from build123d import *

# Parameters (mm, degrees)
SKETCH1_R           = 6.33
BOSS_EXTRUDE1_DEPTH = 1.5
SKETCH2_R           = 20.2
BOSS_EXTRUDE2_DEPTH = 71
SKETCH6_R           = 6
BOSS_EXTRUDE4_DEPTH = 3
SKETCH7_R           = 2
BOSS_EXTRUDE5_DEPTH = 9
SKETCH8_R           = 1.65
CUT_EXTRUDE1_DEPTH  = 4


with BuildPart() as part:
    # Sketch1 → Boss-Extrude1 (new body)
    with BuildSketch(Plane.XY):
        Circle(SKETCH1_R)
    extrude(amount=BOSS_EXTRUDE1_DEPTH)

    # Sketch2 → Boss-Extrude2 (add)
    with BuildSketch(Plane.XY):
        Circle(SKETCH2_R)
    extrude(amount=-BOSS_EXTRUDE2_DEPTH)

    # Sketch6 → Boss-Extrude4 (add)
    with BuildSketch(Plane(origin=(0, 0, -71), x_dir=(-1, 0, 0), z_dir=(0, 0, -1))):
        Circle(SKETCH6_R)
    extrude(amount=BOSS_EXTRUDE4_DEPTH)

    # Sketch7 → Boss-Extrude5 (add)
    with BuildSketch(Plane(origin=(0, 0, -74), x_dir=(-1, 0, 0), z_dir=(0, 0, -1))):
        Circle(SKETCH7_R)
    extrude(amount=BOSS_EXTRUDE5_DEPTH)

    # Sketch8 → Cut-Extrude1 (cut)
    with BuildSketch(Plane(origin=(0, 0, -71), x_dir=(-1, 0, 0), z_dir=(0, 0, -1))):
        with Locations((-12.5, 0)):
            Circle(SKETCH8_R)
        with Locations((12.5, 0)):
            Circle(SKETCH8_R)
    extrude(amount=-CUT_EXTRUDE1_DEPTH, mode=Mode.SUBTRACT)


solid = part.part
Can you work these out from the model? Positions are in its coordinate system, mm. A direction names the side the tool comes from. Give positions to 0.01 mm unless a question says otherwise; leave off trailing zeros. Order: outer loops, then holes, each group sorted by start corner. A loop starts at its lowest first (then second) coordinate and runs counter-clockwise, first axis right, second up. Notation, with made-up numbers: M -16,75 L 4,75 A19 cw 4,89 Z; hole C 21.25,16 d3. An arc over 180 degrees is marked long. Use a Markdown table: item, result. Add a question column.
Item 1: Suppose I cut it at C-C (z = -52). List the corners of the cut face in (x, y) for me, then the cut area to 3 significant figures.
Item 2: Will these pins go through, and if not, where does the flat tip stop? pin 1 (12 mm diameter, centred on x = 7.5, y = 2, fed in from -Z); pin 2 (3 mm diameter, centred on x = -12.5, y = 0, fed in from +Z); pin 3 (4 mm diameter, centred on x = -1.5, z = -70, fed in from +Y); pin 4 (8 mm diameter, centred on y = -6.5, z = -69.5, fed in from -X).
Item 3: If I drill on L1, parallel to Z at x = 0, y = 15.5; L2, parallel to Y at x = 12.5, z = -68.85; L3, parallel to Y at x = -10, z = -59.5, over which ranges is the centre line in solid material (lowest first)? Write a range as [from, to].
Item 4: Suppose I cut it at B-B (y = 0). List the corners of the cut face in (x, z) for me, then the cut area to 3 significant figures.
Item 5: We'd pull the mould along X, two halves only. Please class faces 1 (the flat face through (-3, 0, -74)), 2 (the cylindrical face through (6, 0, -72)), 3 (the cylindrical face through (10.976, -0.632, -69.028)): +X half, -X half, draft (parallel to the pull), parting line (faces both ways), or undercut.
Item 6: Suppose I cut it at A-A (x = 0). List the corners of the cut face in (y, z) for me.
Item 7: For faces 4 (the flat face through (-5, 5, 0)), 5 (the flat face through (0, 0, -83)), 6 (the flat face through (13, 0, -67)), which set-ups out of +Z, -Z, +X, -X, +Y, -Y let a thin tool reach every point of the face, with its end or its side?
Item 8: Suppose I cut it at D-D (x = 12.5). List the corners of the cut face in (y, z) for me, then the cut area to 3 significant figures.
Answer sheet:
| question | item | result |
|---|---|---|
| 1 | outline | C 0,0 d40.4 |
| 1 | area | 1,280 mm² |
| 2 | pin 1 | stops at z = -83 |
| 2 | pin 2 | stops at z = 0 |
| 2 | pin 3 | stops at y = 20.2 |
| 2 | pin 4 | stops at x = -20.04 |
| 3 | L1 | z = [-71, 0] |
| 3 | L2 | y = [-15.87, -1.65], [1.65, 15.87] |
| 3 | L3 | y = [-17.55, 17.55] |
| 4 | outline | M -20.2,-71 L -14.15,-71 L -14.15,-67 L -10.85,-67 L -10.85,-71 L -6,-71 L -6,-74 L -2,-74 L -2,-83 L 2,-83 L 2,-74 L 6,-74 L 6,-71 L 10.85,-71 L 10.85,-67 L 14.15,-67 L 14.15,-71 L 20.2,-71 L 20.2,0 L 6.33,0 L 6.33,1.5 L -6.33,1.5 L -6.33,0 L -20.2,0 Z |
| 4 | area | 2,930 mm² |
| 5 | face 1 | draft |
| 5 | face 2 | parting line |
| 5 | face 3 | undercut |
| 6 | outline | M -20.2,-71 L -6,-71 L -6,-74 L -2,-74 L -2,-83 L 2,-83 L 2,-74 L 6,-74 L 6,-71 L 20.2,-71 L 20.2,0 L 6.33,0 L 6.33,1.5 L -6.33,1.5 L -6.33,0 L -20.2,0 Z |
| 7 | face 4 | +Z |
| 7 | face 5 | -Z, +X, -X, +Y, -Y |
| 7 | face 6 | -Z |
| 8 | outline | M -15.87,-71 L -1.65,-71 L -1.65,-67 L 1.65,-67 L 1.65,-71 L 15.87,-71 L 15.87,0 L -15.87,0 Z |
| 8 | area | 2,240 mm² |
